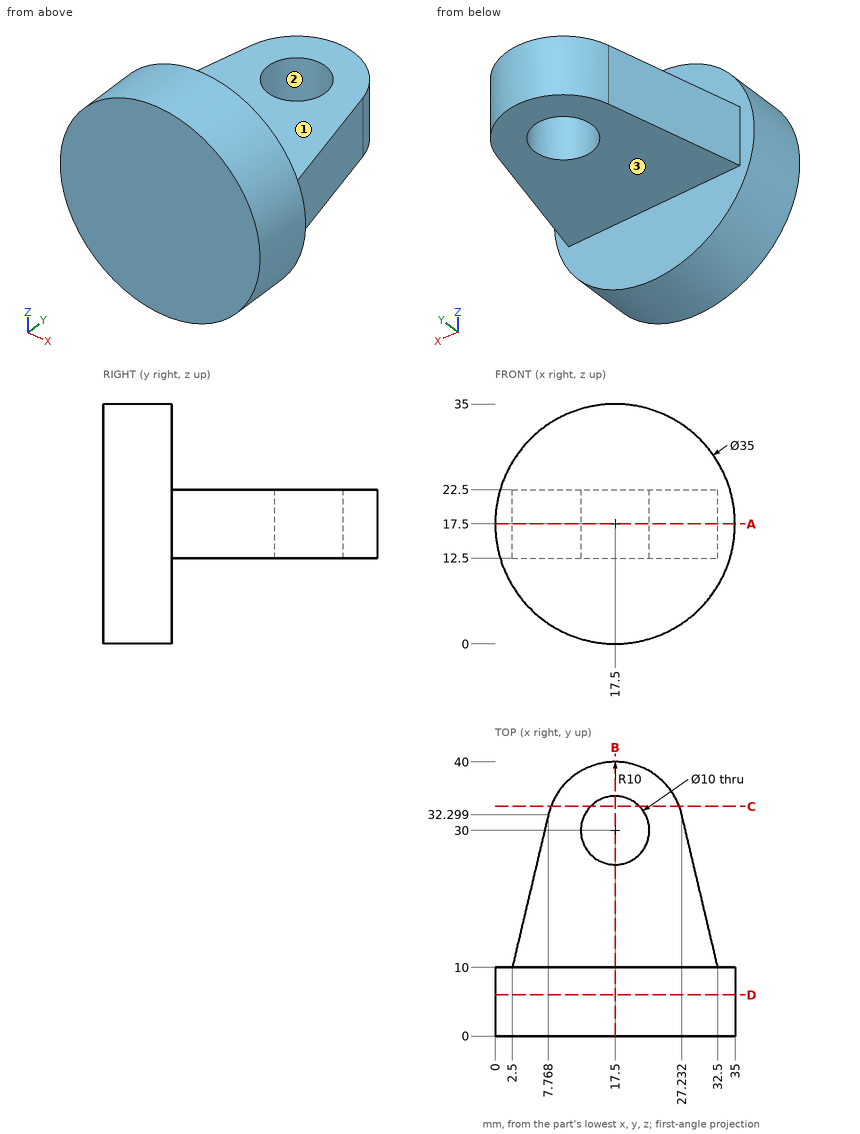
Can you work these out from the drawing? Everything is in mm from the part's minimum corner. A direction names the side the tool comes from. Coordinates: 2 decimals unless noted, no trailing zeros. Loops run counter-clockwise (first coordinate to the right, second up) from the corner with the lowest first, then second, coordinate; pieces in that order, holes last. Notation, with made-up numbers: (63, 46.25) - (91, 46.25) arc R34 ccw to (91, 78.25) - close; hole circle Ø7 at (63.5, -36.5). An arc over 180 degrees is marked (long way). Use a Markdown table: item, result.
Item 1: I want a section at B-B on x = 17.5. Please give me the cut outline in (y, z), and give its area (3 significant figures).
Numbers:
| item | result |
|---|---|
| outline | (0, 0) - (10, 0) - (10, 12.5) - (25, 12.5) - (25, 22.5) - (10, 22.5) - (10, 35) - (0, 35) - close; (35, 12.5) - (40, 12.5) - (40, 22.5) - (35, 22.5) - close |
| area | 550 mm2 |
Item 2: I want a section at C-C on y = 33.5. Please give me the cut outline in (x, z), and give its area (3 significant figures).
Numbers:
| item | result |
|---|---|
| outline | (8.13, 12.5) - (13.93, 12.5) - (13.93, 22.5) - (8.13, 22.5) - close; (21.07, 12.5) - (26.87, 12.5) - (26.87, 22.5) - (21.07, 22.5) - close |
| area | 116 mm2 |
Item 3: If I drill on probe 1 along Y at (x, z) = (17.5, 17.5); probe 2 along Z at (x, y) = (4, 16); probe 3 along Y at (x, z) = (14.5, 7), over which ranges is the centre line in solid material (lowest first)? Write a range as from..to.
Numbers:
| item | result |
|---|---|
| probe 1 | y = 0..25, 35..40 |
| probe 2 | z = 12.5..22.5 |
| probe 3 | y = 0..10 |
Item 4: I want a section at D-D on y = 6. Please give me the cut outline in (x, z).
Numbers:
| item | result |
|---|---|
| outline | circle Ø35 at (17.5, 17.5) |
Item 5: For the marked faces 1, 2 and 3, which set-ups out of +Z, -Z, +X, -X, +Y, -Y let a thin tool reach every point of the face, with its end or its side?
Numbers:
| item | result |
|---|---|
| face 1 | +Z, +X, -X, +Y |
| face 2 | +Z, -Z |
| face 3 | -Z, +X, -X, +Y |
Item 6: I want a section at A-A on z = 17.5. Please give me the cut outline in (x, y).
Numbers:
| item | result |
|---|---|
| outline | (0, 0) - (35, 0) - (35, 10) - (32.5, 10) - (27.23, 32.3) arc R10 ccw to (7.77, 32.3) - (2.5, 10) - (0, 10) - close; hole circle Ø10 at (17.5, 30) |
Item 7: Will these pins go through, and if not, where does the flat tip stop? pin 1 (4 mm diameter, centred on x = 25, y = 33.5, fed in from +Z); pin 2 (3 mm diameter, centred on y = 33.5, z = 16, fed in from -X); pin 3 (9 mm diameter, centred on x = 17.5, y = 30, fed in from +Z); pin 4 (4 mm diameter, centred on y = 16.5, z = 22, fed in from -X).
Numbers:
| item | result |
|---|---|
| pin 1 | stops at z = 22.5 |
| pin 2 | stops at x = 7.7 |
| pin 3 | passes through |
| pin 4 | stops at x = 3.56 |
